```python
from build123d import *

# Parameters (mm, degrees)
BOSS_EXTRUDE1_DEPTH = 57
SKETCH2_R           = 2.25
CUT_EXTRUDE1_DEPTH  = 92.940197955
SKETCH3_R           = 1.7
SKETCH3_R_2         = 6.25
CUT_EXTRUDE2_DEPTH  = 52


with BuildPart() as part:
    # Sketch1 → Boss-Extrude1 (new body)
    with BuildSketch(Plane(origin=(0, 0, 0), x_dir=(1, 0, 0), z_dir=(0, 1, 0))):
        with BuildLine():
            Line((-2, 0), (-2, 49))
            ThreePointArc((-2, 49), (-1.121320344, 51.121320344), (1, 52))
            Line((1, 52), (45, 52))
            ThreePointArc((45, 52), (47.121320344, 51.121320344), (48, 49))
            Line((48, 49), (48, 0))
            Line((48, 0), (46, 0))
            Line((46, 0), (46, 49))
            ThreePointArc((46, 49), (45.707106781, 49.707106781), (45, 50))
            Line((45, 50), (1, 50))
            ThreePointArc((1, 50), (0.292893219, 49.707106781), (0, 49))
            Line((0, 49), (0, 0))
            Line((0, 0), (-2, 0))
        make_face()
    extrude(amount=BOSS_EXTRUDE1_DEPTH)

    # Sketch2 → Cut-Extrude1 (cut, through all)
    with BuildSketch(Plane(origin=(48, 0, 0), x_dir=(0, 0, -1), z_dir=(1, 0, 0))):
        with Locations((6, 51)):
            Circle(SKETCH2_R)
        with Locations((44, 51)):
            Circle(SKETCH2_R)
        with Locations((6, 6)):
            Circle(SKETCH2_R)
        with Locations((44, 6)):
            Circle(SKETCH2_R)
    extrude(amount=-CUT_EXTRUDE1_DEPTH, mode=Mode.SUBTRACT)

    # Sketch3 → Cut-Extrude2 (cut)
    with BuildSketch(Plane(origin=(0, 0, -52), x_dir=(-1, 0, 0), z_dir=(0, 0, -1))):
        with Locations((-38.5, 28.5)):
            Circle(SKETCH3_R)
        with Locations((-30.75, 41.923393759)):
            Circle(SKETCH3_R)
        with Locations((-15.25, 41.923393759)):
            Circle(SKETCH3_R)
        with Locations((-7.5, 28.5)):
            Circle(SKETCH3_R)
        with Locations((-15.25, 15.076606241)):
            Circle(SKETCH3_R)
        with Locations((-30.75, 15.076606241)):
            Circle(SKETCH3_R)
        with Locations((-23, 35.5)):
            Circle(SKETCH3_R_2)
    extrude(amount=-CUT_EXTRUDE2_DEPTH, mode=Mode.SUBTRACT)


solid = part.part
```
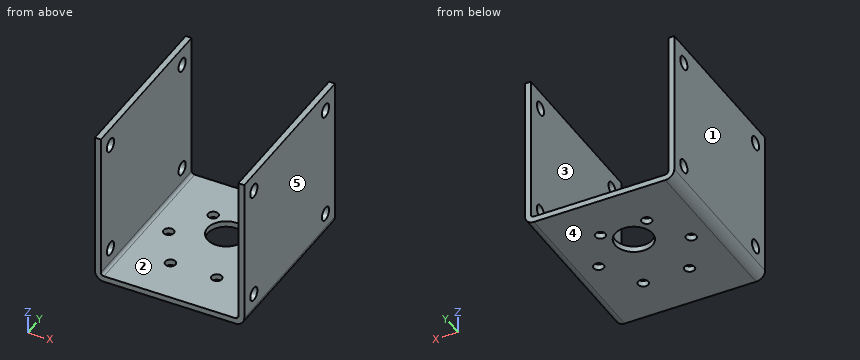
Geometry check sheet. Reference: the model listing, model coordinates, mm. Face numbers are marked on the shaded views. A direction names the side the tool comes from. Round coordinates to 2 decimals unless told otherwise and drop trailing zeros. Order: outer loops, then holes, each group sorted by start corner. A loop starts at its lowest first (then second) coordinate and runs counter-clockwise, first axis right, second up. Notation, with made-up numbers: (20.25, 55) - (69.25, 55) arc R14 cw to (69.25, 68) - close; hole circle Ø9 at (87.5, -17). An arc over 180 degrees is marked (long way). Use a Markdown table: item, result. Add a question column.
1) Section check B-B (y = 35.5). Record the cut outline in (x, z), then the cut area to 3 significant figures.
2) Gauge pin test, flat end, axial feed: P1, Ø8, axis at x = 26.5, y = 14, coming from the +Z side. Record the tip position at first contact, or that the pin passes through.
3) Thickness scan on line 1 along Y through (x, z) = (47, -6); line 2 along Y through (x, z) = (15.25, -51.4); line 3 along X through (y, z) = (41.5, -41). Record the ranges inside material, lowest first.
4) Mould release check, pull along X, two halves, no side actions. Record for the marked faces 3, 4 and 5: released by +X, released by -X, zero draft, split by the parting line, or undercut.
5) Set-up check for the marked faces 1 and 2: record each of +Z, -Z, +X, -X, +Y, -Y from which the full face is reachable in a straight line by a thin tool's end or side.
6) Section check D-D (z = -44). Record the cut outline in (x, y).
7) Section check C-C (x = 38.5). Record the cut outline in (y, z), then the cut area to 3 significant figures.
8) Section check A-A (z = -3). Record the cut outline in (x, y), then the cut area to 3 significant figures.
Established:
| question | item | result |
|---|---|---|
| 1 | outline | (-2, -49) arc R3 ccw to (1, -52) - (16.75, -52) - (16.75, -50) - (1, -50) arc R1 cw to (0, -49) - (0, 0) - (-2, 0) - close; (29.25, -52) - (45, -52) arc R3 ccw to (48, -49) - (48, 0) - (46, 0) - (46, -49) arc R1 cw to (45, -50) - (29.25, -50) - close |
| 1 | area | 272 mm2 |
| 2 | P1 | z = -50 |
| 3 | line 1 | 0 to 3.75, 8.25 to 48.75, 53.25 to 57 |
| 3 | line 2 | 0 to 13.38, 16.78 to 40.22, 43.62 to 57 |
| 3 | line 3 | -2 to 0, 46 to 48 |
| 4 | face 3 | undercut |
| 4 | face 4 | zero draft |
| 4 | face 5 | released by +X |
| 5 | face 1 | +Z, -Z, -X, +Y, -Y |
| 5 | face 2 | +Z, +Y, -Y |
| 6 | outline | (-2, 0) - (0, 0) - (0, 3.75) - (-2, 3.75) - close; (-2, 8.25) - (0, 8.25) - (0, 48.75) - (-2, 48.75) - close; (-2, 53.25) - (0, 53.25) - (0, 57) - (-2, 57) - close; (46, 0) - (48, 0) - (48, 3.75) - (46, 3.75) - close; (46, 8.25) - (48, 8.25) - (48, 48.75) - (46, 48.75) - close; (46, 53.25) - (48, 53.25) - (48, 57) - (46, 57) - close |
| 7 | outline | (0, -52) - (26.8, -52) - (26.8, -50) - (0, -50) - close; (30.2, -52) - (57, -52) - (57, -50) - (30.2, -50) - close |
| 7 | area | 107 mm2 |
| 8 | outline | (-2, 0) - (0, 0) - (0, 57) - (-2, 57) - close; (46, 0) - (48, 0) - (48, 57) - (46, 57) - close |
| 8 | area | 228 mm2 |
